Could you check a few things on this model? Use its own coordinates, in mm. Face numbers are marked on the shaded views. A direction names the side the tool comes from. Coordinates: 2 decimals unless noted, no trailing zeros. Order: outer loops, then holes, each group sorted by start corner. A loop starts at its lowest first (then second) coordinate and runs counter-clockwise, first axis right, second up. Notation, with made-up numbers: M 63.25,75 L 115.25,75 A16 cw 115.25,101 Z; hole C 79.25,-9 d1. An arc over 180 degrees is marked long. Write item = value, one per line. Start each with the question number.
from build123d import *

# Parameters (mm, degrees)
SKETCH1_W           = 20
SKETCH1_H           = 19.6
SKETCH1_R           = 1
BOSS_EXTRUDE1_DEPTH = 1
SKETCH2_W           = 20
SKETCH2_H           = 1
BOSS_EXTRUDE2_DEPTH = 30
SKETCH3_W           = 20
SKETCH3_H           = 1
BOSS_EXTRUDE3_DEPTH = 10


with BuildPart() as part:
    # Sketch1 → Boss-Extrude1 (new body)
    with BuildSketch(Plane.XY):
        Rectangle(SKETCH1_W, SKETCH1_H)
        with Locations((-8.256, 0)):
            Circle(SKETCH1_R, mode=Mode.SUBTRACT)
        with Locations((8.256, 0)):
            Circle(SKETCH1_R, mode=Mode.SUBTRACT)
    extrude(amount=BOSS_EXTRUDE1_DEPTH)

    # Sketch2 → Boss-Extrude2 (add)
    with BuildSketch(Plane.XY.offset(1)):
        with Locations((0, -9.3)):
            Rectangle(SKETCH2_W, SKETCH2_H)
    extrude(amount=BOSS_EXTRUDE2_DEPTH)

    # Sketch3 → Boss-Extrude3 (add)
    with BuildSketch(Plane(origin=(0, -8.8, 0), x_dir=(1, 0, 0), z_dir=(0, 1, 0))):
        with Locations((0, -30.5)):
            Rectangle(SKETCH3_W, SKETCH3_H)
    extrude(amount=BOSS_EXTRUDE3_DEPTH)


solid = part.part
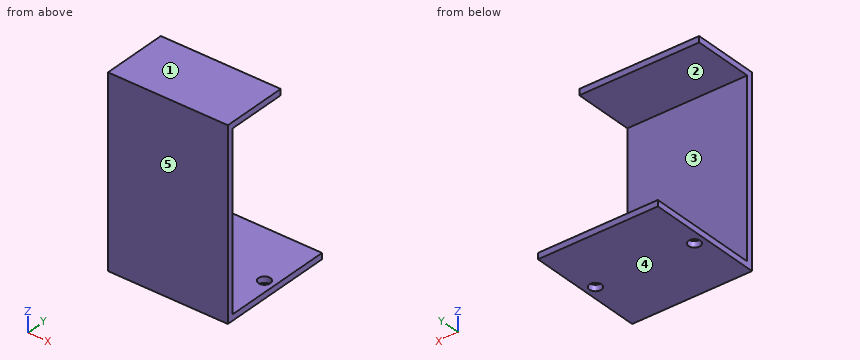
(1) Imagine slicing it at B-B on y = -6.25. List the corners of the cut face in (x, z) for me, plus the area to 3 significant figures.
(2) Imagine slicing it at D-D on x = 3.5. List the corners of the cut face in (y, z) for me.
(3) Please list where these lines run through material, in increasing order: probe 1 along Z at (x, y) = (5.5, -0.25); probe 2 along Y at (x, z) = (1.5, 3.5); probe 3 along Z at (x, y) = (-1.75, 2). Write a range as from..to.
(4) Imagine slicing it at A-A on y = 0. List the corners of the cut face in (x, z) for me, plus the area to 3 significant figures.
(5) Imagine slicing it at C-C on x = 8.75. List the corners of the cut face in (y, z) for me.
(6) Will these pins go through, and if not, where does the flat tip stop? P1, Ø5, axis at x = -3, z = 6.5, coming from the +Y side; P2, Ø0.8, axis at x = -2.5, z = 30.5, coming from the +Y side; P3, Ø5.5, axis at x = 1, y = 2, coming from the +Z side; P4, Ø1.2, axis at x = -8.256, y = 0, coming from the -Z side.
(7) Thinking about a two-plate mould opening in Z: for the marked faces 3, 4 and 5, which applies, released by +Z, released by -Z, zero draft, split by the parting line, or undercut?
(8) For the marked faces 1 and 2, which set-ups out of +Z, -Z, +X, -X, +Y, -Y let a thin tool reach every point of the face, with its end or its side?
Response:
q1.outline = M -10,0 L 10,0 L 10,1 L -10,1 Z; M -10,30 L 10,30 L 10,31 L -10,31 Z
q1.area = 40.0 mm2
q2.outline = M -9.8,0 L 9.8,0 L 9.8,1 L -8.8,1 L -8.8,30 L 1.2,30 L 1.2,31 L -9.8,31 Z
q3.probe_1 = 0..1, 30..31
q3.probe_2 = -9.8..-8.8
q3.probe_3 = 0..1
q4.outline = M -10,0 L -9.26,0 L -9.26,1 L -10,1 Z; M -10,30 L 10,30 L 10,31 L -10,31 Z; M -7.26,0 L 7.26,0 L 7.26,1 L -7.26,1 Z; M 9.26,0 L 10,0 L 10,1 L 9.26,1 Z
q4.area = 36.0 mm2
q5.outline = M -9.8,0 L -0.87,0 L -0.87,1 L -8.8,1 L -8.8,30 L 1.2,30 L 1.2,31 L -9.8,31 Z; M 0.87,0 L 9.8,0 L 9.8,1 L 0.87,1 Z
q6.P1 = -8.8
q6.P2 = 1.2
q6.P3 = 31
q6.P4 = 30
q7.face_3 = undercut
q7.face_4 = released by -Z
q7.face_5 = zero draft
q8.face_1 = +Z, +X, -X, +Y, -Y
q8.face_2 = +X, -X, +Y
